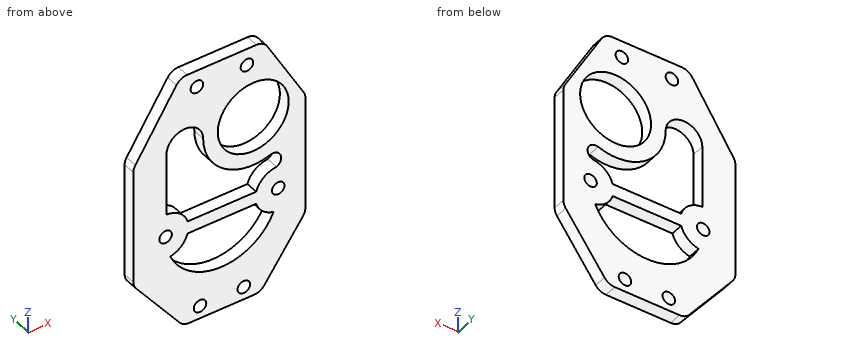
from build123d import *

# Parameters (mm, degrees)
SKETCH1_R          = 8.5
SKETCH1_R_2        = 1.5
BASE_FLANGE1_DEPTH = 3
L_EK1_SCALE        = 2


# Sheet-metal steps are written as plain solids
with BuildPart() as part:
    # Sketch1 → Base-Flange1 (new body)
    with BuildSketch(Plane(origin=(0, 0, 0), x_dir=(1, 0, 0), z_dir=(0, 1, 0))):
        with BuildLine():
            Line((19.609421573, -14.059417906), (10.862109445, -29.480175346))
            ThreePointArc((10.862109445, -29.480175346), (9.762567662, -30.59234701), (8.252687872, -31))
            Line((8.252687872, -31), (-8.352599575, -31))
            ThreePointArc((-8.352599575, -31), (-9.796606082, -30.629609326), (-10.884048227, -29.609896806))
            Line((-10.884048227, -29.609896806), (-20.742852548, -14.107625594))
            ThreePointArc((-20.742852548, -14.107625594), (-21.091885276, -13.336076582), (-21.211403896, -12.497728788))
            Line((-21.211403896, -12.497728788), (-21.211403896, 14.839305313))
            ThreePointArc((-21.211403896, 14.839305313), (-21.044943633, 15.824725306), (-20.564035521, 16.700789784))
            Line((-20.564035521, 16.700789784), (-10.150833328, 29.861484472))
            ThreePointArc((-10.150833328, 29.861484472), (-9.105019706, 30.700412322), (-7.798201703, 31))
            Line((-7.798201703, 31), (7.702138241, 31))
            ThreePointArc((7.702138241, 31), (9.077698333, 30.666052219), (10.147014932, 29.738556288))
            Line((10.147014932, 29.738556288), (19.444876691, 16.663267527))
            ThreePointArc((19.444876691, 16.663267527), (19.857851472, 15.837226972), (20, 14.924711239))
            Line((20, 14.924711239), (20, -12.57924256))
            ThreePointArc((20, -12.57924256), (19.900712388, -13.344662472), (19.609421573, -14.059417906))
        make_face()
        with Locations(Location((7.5, -13.4, 0), (0, 0, 270))):
            Circle(SKETCH1_R, mode=Mode.SUBTRACT)
        with Locations(Location((6, -27, 0), (0, 0, 270))):
            Circle(SKETCH1_R_2, mode=Mode.SUBTRACT)
        with Locations(Location((-6, -27, 0), (0, 0, 270))):
            Circle(SKETCH1_R_2, mode=Mode.SUBTRACT)
        with Locations(Location((5.25, 27.940782939, 0), (0, 0, 270))):
            Circle(SKETCH1_R_2, mode=Mode.SUBTRACT)
        with Locations(Location((-5.25, 27.940782939, 0), (0, 0, 270))):
            Circle(SKETCH1_R_2, mode=Mode.SUBTRACT)
        with Locations(Location((13.5, 7.05, 0), (0, 0, 270))):
            Circle(SKETCH1_R_2, mode=Mode.SUBTRACT)
        with Locations(Location((-13.5, 7.05, 0), (0, 0, 270))):
            Circle(SKETCH1_R_2, mode=Mode.SUBTRACT)
        with BuildLine():
            Line((-13.281403896, 0), (-13.281403896, 1.567980996))
            ThreePointArc((-13.281403896, 1.567980996), (-10.106558233, 2.738982767), (-8.222660082, 5.55))
            Line((-8.222660082, 5.55), (8.208497378, 5.55))
            ThreePointArc((8.208497378, 5.55), (10.031018679, 2.781959631), (13.113110627, 1.563624456))
            ThreePointArc((13.113110627, 1.563624456), (14.07117407, -0.953003234), (11.655254401, -2.142386538))
            ThreePointArc((11.655254401, -2.142386538), (0.639353267, -3.554619032), (-4.5, -13.4))
            ThreePointArc((-4.5, -13.4), (-8.890701948, -17.790701948), (-13.281403896, -13.4))
            Line((-13.281403896, -13.4), (-13.281403896, 0))
        make_face(mode=Mode.SUBTRACT)
        with BuildLine():
            Line((-8.222660082, 8.55), (8.208497378, 8.55))
            ThreePointArc((8.208497378, 8.55), (9.751572067, 11.074833914), (12.37962963, 12.434679214))
            ThreePointArc((12.37962963, 12.434679214), (-0.006957749, 20.549998207), (-12.385173459, 12.42191571))
            ThreePointArc((-12.385173459, 12.42191571), (-9.763306163, 11.067142739), (-8.222660082, 8.55))
        make_face(mode=Mode.SUBTRACT)
    extrude(amount=BASE_FLANGE1_DEPTH)


with BuildPart() as part_1:
    # Ölçek1: scaled about (-1.130925292, 1.5, -0.876080417)
    add(part.part.scale(L_EK1_SCALE).moved(Location((1.130925292, -1.5, 0.876080417))))


solid = part_1.part
Verification items for the finished model (mm, model axes). Round coordinates to 2 decimals unless told otherwise and drop trailing zeros. Loops run counter-clockwise (first coordinate to the right, second up) from the corner with the lowest first, then second, coordinate; pieces in that order, holes last. Notation, with made-up numbers: (-26, -37) - (1, -37) arc R23 cw to (1, -26) - close; hole circle Ø8 at (-27.5, -33). An arc over 180 degrees is marked (long way). Write item = value, one per line.
Q1. Sectioned sample at A-A on x = 7. Record the boundary of the cut face in (y, z), plus the area to 3 significant figures.
Here are the results:
outline = (-1.5, -61.12) - (4.5, -61.12) - (4.5, -39.58) - (-1.5, -39.58) - close; (-1.5, -16.22) - (4.5, -16.22) - (4.5, -10.22) - (-1.5, -10.22) - close; (-1.5, 5.48) - (4.5, 5.48) - (4.5, 13.34) - (-1.5, 13.34) - close; (-1.5, 42.02) - (4.5, 42.02) - (4.5, 62.88) - (-1.5, 62.88) - close
area = 338 mm^2
Q2. Sectioned sample at D-D on y = 1.45. State how many separate pieces and enclosed holes the cut face has, plus the area to 3 significant figures.
Here are the results:
separate_pieces = 1
enclosed_holes = 9
area = 5,520 mm^2
Q3. Material ranges on L1, parallel to X at y = 2.35, z = -14; L2, parallel to Z at x = -15, y = 2.2; L3, parallel to Z at x = 8, y = 0.95, recorded low to high.
Here are the results:
L1 = -41.29 to -28.77, -22.97 to 25.23, 31.03 to 41.13
L2 = -61.1 to -34.88, -16.22 to -10.22, 36.3 to 62.88
L3 = -61.12 to -39.34, -16.22 to -10.22, 5.1 to 12.75, 42.61 to 62.88
Q4. Depth check by flat-ended pin: pin 1 (5 mm diameter, centred on x = -9.37, z = -55.01, fed in from +Y); pin 2 (1 mm diameter, centred on x = -20, y = 1.5, fed in from -Z). Enter the tip coordinate at first touch or a pass-through.
Here are the results:
pin_1 = through
pin_2 = -58.43
Q5. Sectioned sample at C-C on x = -4. Record the boundary of the cut face in (y, z).
Here are the results:
outline = (-1.5, -61.12) - (4.5, -61.12) - (4.5, -39.73) - (-1.5, -39.73) - close; (-1.5, -16.22) - (4.5, -16.22) - (4.5, -10.22) - (-1.5, -10.22) - close; (-1.5, 14.61) - (4.5, 14.61) - (4.5, 62.88) - (-1.5, 62.88) - close
Q6. Sectioned sample at B-B on z = -14.5. Record the boundary of the cut face in (x, y), plus the area to 3 significant figures.
Here are the results:
outline = (-41.29, -1.5) - (-28.58, -1.5) - (-28.58, 4.5) - (-41.29, 4.5) - close; (-23.15, -1.5) - (25.42, -1.5) - (25.42, 4.5) - (-23.15, 4.5) - close; (30.85, -1.5) - (41.13, -1.5) - (41.13, 4.5) - (30.85, 4.5) - close
area = 429 mm^2
